Build history of the part. All positions in model axes, mm. Coordinates: 2 decimals unless noted, no trailing zeros. Loops run counter-clockwise (first coordinate to the right, second up) from the corner with the lowest first, then second, coordinate; pieces in that order, holes last. Notation, with made-up numbers: (75, -7) - (109, -7) arc R33 cw to (109, 21) - close; hole circle Ø2 at (-14.75, -38.75). An arc over 180 degrees is marked (long way). One line per item, written item: value.
```python
from build123d import *

# Parameters (mm, degrees)
SKETCH_1_W         = 20
SKETCH_1_H         = 40
SKETCH_1_R         = 3.25
EXTRUDE_1_DEPTH    = 6
HOLE_WIZARD_M6_1_D = 5


with BuildPart() as part:
    # 草图1 → 凸台-拉伸1 (new body)
    with BuildSketch(Plane(origin=(0, 0, 0), x_dir=(1, 0, 0), z_dir=(0, 1, 0))):
        with Locations((10, 20)):
            Rectangle(SKETCH_1_W, SKETCH_1_H)
        with Locations(Location((10, 30, 0), (0, 0, 270))):
            Circle(SKETCH_1_R, mode=Mode.SUBTRACT)
        with Locations(Location((10, 10, 0), (0, 0, 270))):
            Circle(SKETCH_1_R, mode=Mode.SUBTRACT)
    extrude(amount=EXTRUDE_1_DEPTH)

    # M6 螺纹孔1 (through all)
    with Locations(Plane(origin=(10, 6, -20), x_dir=(0, 0, 1), z_dir=(0, 1, 0))):
        with Locations((0, 0)):
            Hole(HOLE_WIZARD_M6_1_D / 2)


solid = part.part
```
Item 1: Cut at B-B, the plane y = 1. Write the cut outline in (x, z), then the cut area to 3 significant figures.
Check result:
outline: (0, -40) - (20, -40) - (20, 0) - (0, 0) - close; hole circle Ø6.5 at (10, -30); hole circle Ø6.5 at (10, -10); hole circle Ø5 at (10, -20)
area: 714 mm^2
Item 2: Cut at D-D, the plane z = -30. Write the cut outline in (x, y), then the cut area to 3 significant figures.
Check result:
outline: (0, 0) - (6.75, 0) - (6.75, 6) - (0, 6) - close; (13.25, 0) - (20, 0) - (20, 6) - (13.25, 6) - close
area: 81.0 mm^2
Item 3: Drop a flat-ended pin along its axis: P1, Ø5, axis at x = 10, z = -30, coming from the -Y side. Give the stop position or say it passes through.
Check result:
P1: passes through
Item 4: Cut at A-A, the plane z = -20. Write the cut outline in (x, y).
Check result:
outline: (0, 0) - (7.5, 0) - (7.5, 6) - (0, 6) - close; (12.5, 0) - (20, 0) - (20, 6) - (12.5, 6) - close
Item 5: Probe probe 1 along X at (y, z) = (2, -30); probe 2 along X at (y, z) = (4.3, -20); probe 3 along Z at (x, y) = (10.25, 0.9). List the from-to ranges inside material, lowest first. Write a range as from..to.
Check result:
probe 1: x = 0..6.75, 13.25..20
probe 2: x = 0..7.5, 12.5..20
probe 3: z = -40..-33.24, -26.76..-22.49, -17.51..-13.24, -6.76..0
Item 6: Cut at C-C, the plane x = 10. Write the cut outline in (y, z).
Check result:
outline: (0, -40) - (6, -40) - (6, -33.25) - (0, -33.25) - close; (0, -26.75) - (6, -26.75) - (6, -22.5) - (0, -22.5) - close; (0, -17.5) - (6, -17.5) - (6, -13.25) - (0, -13.25) - close; (0, -6.75) - (6, -6.75) - (6, 0) - (0, 0) - close
Item 7: Pull direction Z, two halves, no side cores. Call faces 1 (the face through (10, 3, 0)), 2 (the face through (10, 0, -25)), 3 (the face through (12.197, 2.958, -12.395)): released by +Z, released by -Z, zero draft, split by the parting line, or undercut.
Check result:
face 1: released by +Z
face 2: zero draft
face 3: undercut
